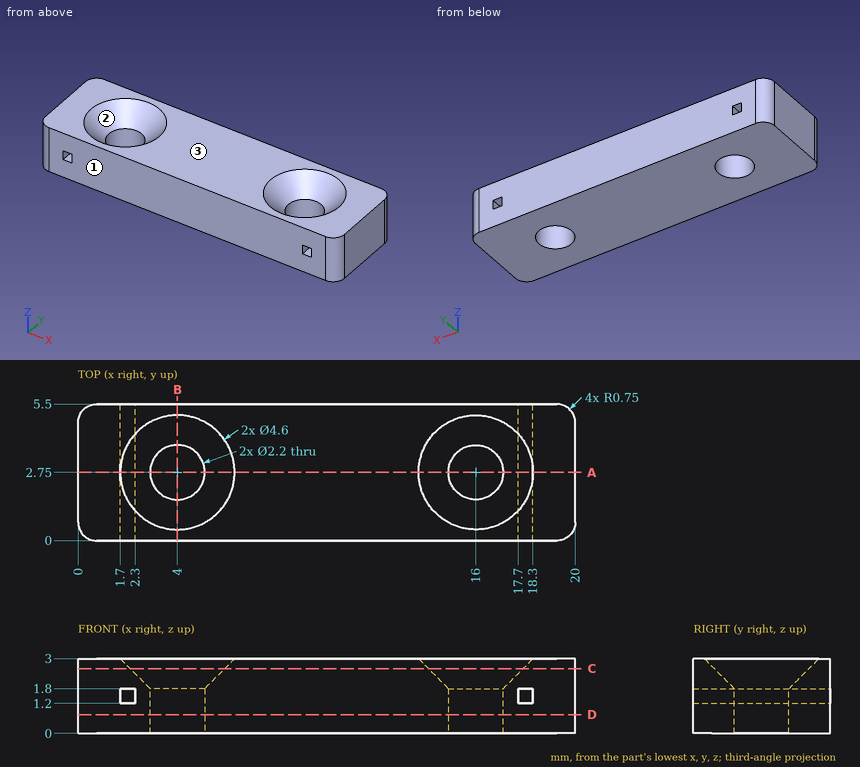
Drawing for the job (mm, zero at the part's lowest x, y, z). Give positions to 0.01 mm unless a question says otherwise; leave off trailing zeros. Loops run counter-clockwise (first coordinate to the right, second up) from the corner with the lowest first, then second, coordinate; pieces in that order, holes last. Notation, with made-up numbers: M -33.75,19.5 L -26.75,19.5 A21 cw -26.75,29.5 Z; hole C -17.75,-22.5 d5. An arc over 180 degrees is marked long. Use one line per item in the form item = value.
Item 1: Slice it at C-C (z = 2.6). List the corners of the cut face in (x, y).
Determined:
outline = M 0,0.75 A0.75 ccw 0.75,0 L 19.25,0 A0.75 ccw 20,0.75 L 20,4.75 A0.75 ccw 19.25,5.5 L 0.75,5.5 A0.75 ccw 0,4.75 Z; hole C 4,2.75 d3.8; hole C 16,2.75 d3.8
Item 2: Slice it at B-B (x = 4). List the corners of the cut face in (y, z), plus the area to 3 significant figures.
Determined:
outline = M 0,0 L 1.65,0 L 1.65,1.8 L 0.45,3 L 0,3 Z; M 3.85,0 L 5.5,0 L 5.5,3 L 5.05,3 L 3.85,1.8 Z
area = 8.46 mm2
Item 3: Flat gauge pin, fed straight in: pin 1 (0.5 mm diameter, centred on x = 18, y = 3.5, fed in from -Z). Where does the tip first touch, or does it go through?
Determined:
pin_1 = 0
Item 4: Drill centre lines: probe 1 along X at (y, z) = (2.7, 1.15); probe 2 along X at (y, z) = (0.9, 2.75); probe 3 along Y at (x, z) = (4, 0.7). Where is each one in solid material? Low to high. Write a range as from..to.
Determined:
probe_1 = 0..2.9, 5.1..14.9, 17.1..20
probe_2 = 0..3.12, 4.88..15.12, 16.88..20
probe_3 = 0..1.65, 3.85..5.5
Item 5: Slice it at D-D (z = 0.75). List the corners of the cut face in (x, y).
Determined:
outline = M 0,0.75 A0.75 ccw 0.75,0 L 19.25,0 A0.75 ccw 20,0.75 L 20,4.75 A0.75 ccw 19.25,5.5 L 0.75,5.5 A0.75 ccw 0,4.75 Z; hole C 4,2.75 d2.2; hole C 16,2.75 d2.2
Item 6: Two-plate mould, pull along Y, no slides. Class the marked faces 1, 2 and 3: pulls with the +Y half, pulls with the -Y half, needs draft (parallel to the pull), parting line crosses it, or undercut.
Determined:
face_1 = pulls with the -Y half
face_2 = undercut
face_3 = needs draft
Item 7: Slice it at A-A (y = 2.75). List the corners of the cut face in (x, z).
Determined:
outline = M 0,0 L 2.9,0 L 2.9,1.8 L 1.7,3 L 0,3 Z; M 5.1,0 L 14.9,0 L 14.9,1.8 L 13.7,3 L 6.3,3 L 5.1,1.8 Z; M 17.1,0 L 20,0 L 20,3 L 18.3,3 L 17.1,1.8 Z; hole M 1.7,1.2 L 2.3,1.2 L 2.3,1.8 L 1.7,1.8 Z; hole M 17.7,1.2 L 18.3,1.2 L 18.3,1.8 L 17.7,1.8 Z
